Could you check a few things on this drawing? It's one solid part, dimensions in mm from its lowest x, y, z. Give positions to 0.01 mm unless a question says otherwise; leave off trailing zeros. Loops run counter-clockwise (first coordinate to the right, second up) from the corner with the lowest first, then second, coordinate; pieces in that order, holes last. Notation, with made-up numbers: M 57.25,83 L 92.25,83 A15 cw 92.25,99 Z; hole C 21.5,5 d9. An arc over 180 degrees is marked long. Answer as a JSON object with one key per item and string values.
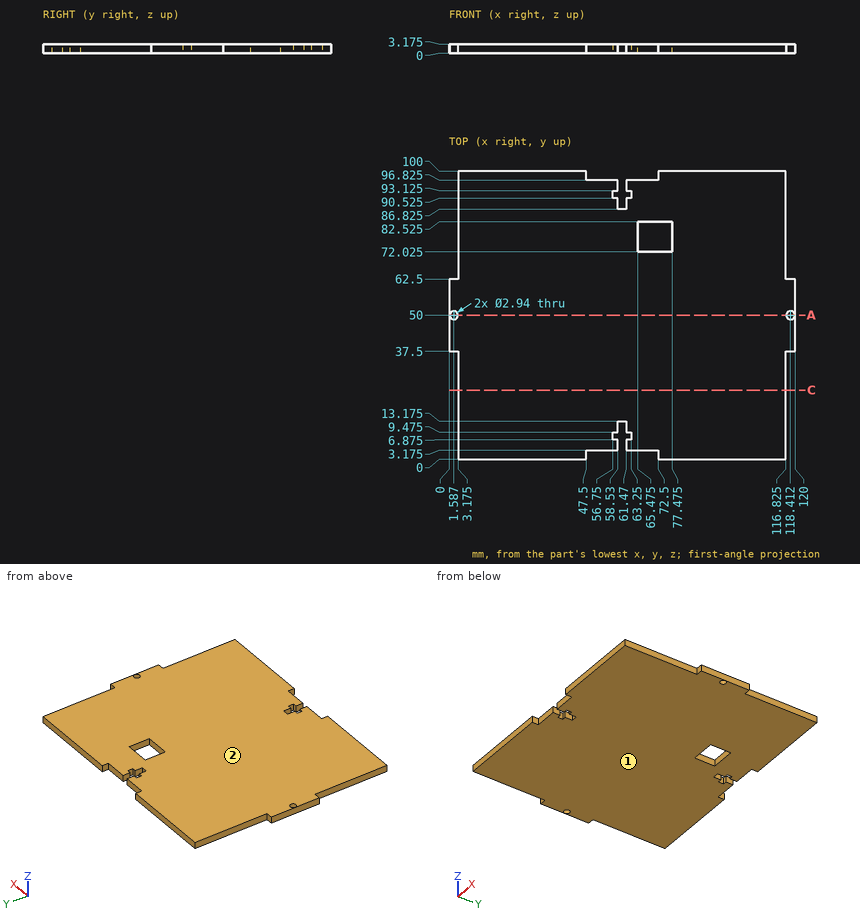
1) If we mould it in two halves opening along Z, with no side actions, what happens to the marked faces 1 and 2? For each: +Z half, -Z half, draft (parallel to the pull), parting line (faces both ways), or undercut.
Answer list:
{"face 1": "-Z half", "face 2": "+Z half"}
2) Suppose I cut it at A-A, the plane y = 50. Give the number of separate pieces and of enclosed holes in the cut face.
Answer list:
{"separate pieces": "3", "enclosed holes": "0"}
3) Will these pins go through, and if not, where does the flat tip stop? pin 1 Ø1.5 at (x, z) = (71, 2) entering from -Y (1 decimal); pin 2 Ø1 at (x, y) = (81, 13.5) entering from -Z; pin 3 Ø0.9 at (x, z) = (57, 1) entering from +Y (1 decimal); pin 4 Ø1 at (y, z) = (2, 2) entering from -X (1 decimal).
Answer list:
{"pin 1": "y = 3.2", "pin 2": "z = 0", "pin 3": "y = 96.8", "pin 4": "x = 3.2"}
4) Please list where these lines run through material, in increasing order: line 1 along Y through (x, z) = (68.5, 1.45) (1 decimal); line 2 along X through (y, z) = (16.5, 1.6) (1 decimal); line 3 along X through (y, z) = (76, 2.9) (1 decimal). Write a range as from..to.
Answer list:
{"line 1": "3.2..72, 82.5..96.8", "line 2": "3.2..116.8", "line 3": "3.2..65.5, 77.5..116.8"}
5) Suppose I cut it at C-C, the plane y = 24. Write out the boundary of the cut face in (x, z) (1 decimal).
Answer list:
{"outline": "M 3.2,0 L 116.8,0 L 116.8,3.2 L 3.2,3.2 Z"}
